The figure shows three views and two pictorial views of one solid part (mm, origin at its lowest corner). Answer the questions. Coordinates: 2 decimals unless noted, no trailing zeros. Write each loop counter-clockwise with the first axis right and the second up, starting at its lowest first coordinate (ties: lowest second). Pieces come first, ordered by that corner, then holes. Notation, with made-up numbers: M 5,26.5 L 56,26.5 A15 cw 56,30.5 Z; hole C 19,22.5 d11. An arc over 180 degrees is marked long. Write item = value, one per line. Start each with the question number.
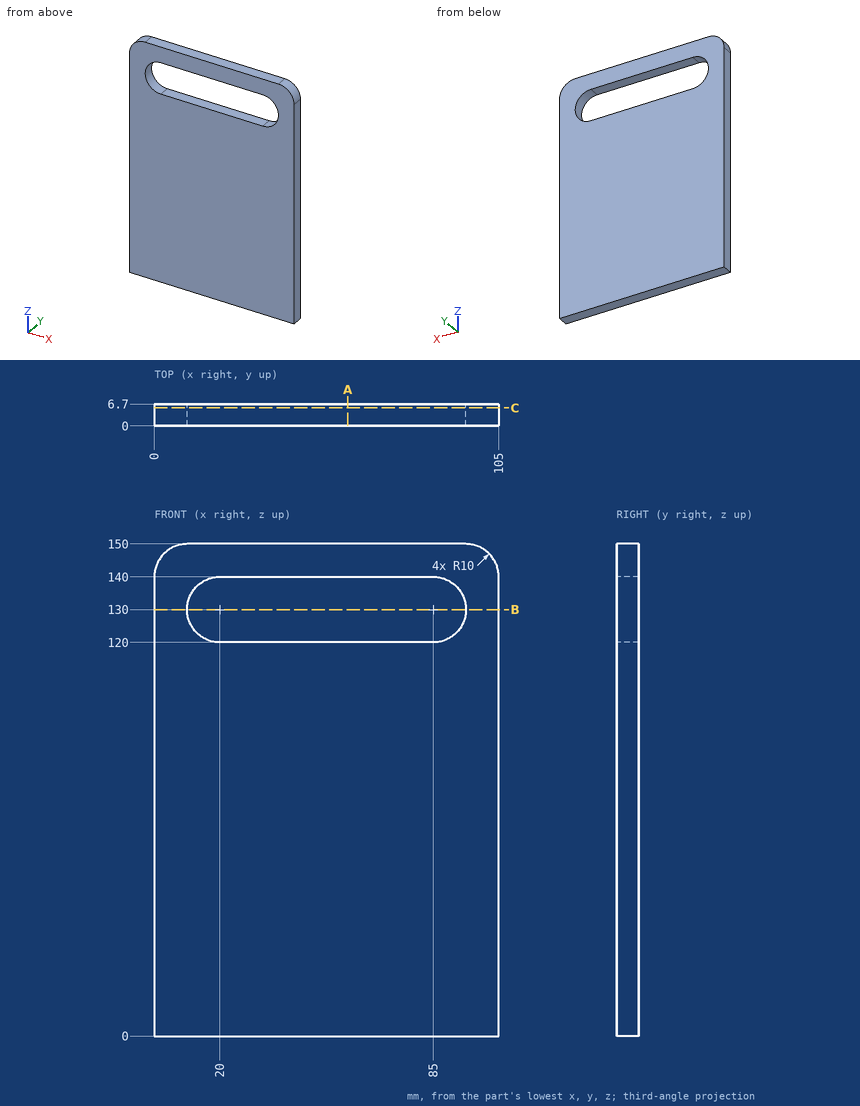
1. The part is cut by section A-A, the plane x = 59. Write down the section's boundary in (y, z), and give its area (3 significant figures).
2. The part is cut by section B-B, the plane z = 130. Write down the section's boundary in (x, y), and give its area (3 significant figures).
3. Straight lines are drawn through the part: L1, parallel to Z at x = 20, y = 5.5; L2, parallel to Z at x = 14, y = 4; L3, parallel to X at y = 0.5, z = 128.5. For each, find the intervals that lie inside material, in ascending order. Write a range as [from, to].
4. The part is cut by section C-C, the plane y = 5.5. Write down the section's boundary in (x, z).
Solution:
q1.outline = M 0,0 L 6.7,0 L 6.7,120 L 0,120 Z; M 0,140 L 6.7,140 L 6.7,150 L 0,150 Z
q1.area = 871 mm^2
q2.outline = M 0,0 L 10,0 L 10,6.7 L 0,6.7 Z; M 95,0 L 105,0 L 105,6.7 L 95,6.7 Z
q2.area = 134 mm^2
q3.L1 = [0, 120], [140, 150]
q3.L2 = [0, 122], [138, 150]
q3.L3 = [0, 10.11], [94.89, 105]
q4.outline = M 0,0 L 105,0 L 105,140 A10 ccw 95,150 L 10,150 A10 ccw 0,140 Z; hole M 20,120 L 85,120 A10 ccw 85,140 L 20,140 A10 ccw Z
